```python
from build123d import *

# Parameters (mm, degrees)
F1_DEPTH = 17.5
F3_DEPTH = 15
F4_R     = 2
F5_SIZE  = 1
F7_DEPTH = 2.5
F8_R     = 1.5
F9_DEPTH = 2.5


with BuildPart() as f1:
    # F0 (on Right) → F1 (new body, symmetric)
    with BuildSketch(Plane.YZ):
        Polygon((-5, -15), (0, -15), (0, 0), (-13.9, 0), (-13.9, -15), (-10.9, -15), (-10.9, -3), (-5, -3), align=None)
    extrude(amount=F1_DEPTH, both=True)

    # F2 (on face) → F3 (join)
    with BuildSketch(Plane.XY):
        with BuildLine():
            Line((0, 0), (3.4641016151, 0))
            ThreePointArc((3.4641016151, 0), (2.2943057454, 5.2766081772), (-3.0641777725, 4.5711504387))
            ThreePointArc((-3.0641777725, 4.5711504387), (-2.940920939, 3.1623183859), (-1.5320888862, 3.2855752194))
            ThreePointArc((-1.5320888862, 3.2855752194), (1.8126155741, 2.8452365235), (0, 0))
        make_face()
        with BuildLine():
            Line((-3.4641016151, 0), (0, 0))
            ThreePointArc((0, 0), (-1, 0.2679491924), (-1.7320508076, 1))
            Line((-1.7320508076, 1), (-3.4641016151, 0))
        make_face()
    extrude(amount=-F3_DEPTH)

    # F4
    f4_edges = [f1.edges().sort_by_distance(p)[0] for p in [
        (3.464102, 0, -7.5),
        (-3.464102, 0, -7.5),
    ]]
    fillet(f4_edges, radius=F4_R)

    # F5
    f5_edges = [f1.edges().sort_by_distance(p)[0] for p in [
        (-17.5, 0, -7.5),
        (17.5, 0, -7.5),
        (-17.5, -13.9, -7.5),
        (17.5, -13.9, -7.5),
    ]]
    chamfer(f5_edges, length=F5_SIZE)

    # F6 (on face) → F7 (cut)
    with BuildSketch(Plane.XZ.offset(5)):
        Polygon((-12.5588457268, -11.7), (-9.4411542732, -11.7), (-7.8823085464, -9), (-9.4411542732, -6.3), (-12.5588457268, -6.3), (-14.1176914536, -9), align=None)
        Polygon((9.4411542732, -11.7), (12.5588457268, -11.7), (14.1176914536, -9), (12.5588457268, -6.3), (9.4411542732, -6.3), (7.8823085464, -9), align=None)
    extrude(amount=-F7_DEPTH, mode=Mode.SUBTRACT)

    # F8 (on face) → F9 (cut, through all)
    with BuildSketch(Plane(origin=(0, 0, 0), x_dir=(-1, 0, 0), z_dir=(0, 1, 0))):
        with Locations((-11, -9)):
            Circle(F8_R)
        with Locations((11, -9)):
            Circle(F8_R)
    extrude(amount=-F9_DEPTH, mode=Mode.SUBTRACT)


solid = f1.part
```
Work out the finished part from the listing and answer in its coordinate system (mm). A direction names the side the tool comes from. Give positions to 0.01 mm unless a question says otherwise; leave off trailing zeros. Write each loop counter-clockwise with the first axis right and the second up, starting at its lowest first coordinate (ties: lowest second). Pieces come first, ordered by that corner, then holes. Notation, with made-up numbers: (37.25, 39) -> (64.25, 39) arc R21 ccw to (64.25, 64) -> close; hole circle Ø11 at (78, -3.75). An arc over 180 degrees is marked (long way). Write each question's results on one line, items separated by ' | '.
1. Straight lines are drawn through the part: L1, parallel to Z at x = -11, y = -1.1; L2, parallel to Y at x = -7.5, z = -7.75; L3, parallel to Y at x = -0.5, z = -6.75. For each, find the intervals that lie inside material, in ascending order.
Data:
L1: -15 to -10.5, -7.5 to 0 | L2: -13.9 to -10.9, -5 to 0 | L3: -13.9 to -10.9, -5 to 0.06, 3.94 to 5.97
2. Find section B-B on z = -13. Determine the outline of the cut face in (x, y), and give its area (3 significant figures).
Data:
outline: (-17.5, -12.9) -> (-16.5, -13.9) -> (16.5, -13.9) -> (17.5, -12.9) -> (17.5, -10.9) -> (-17.5, -10.9) -> close; (-17.5, -5) -> (17.5, -5) -> (17.5, -1) -> (16.5, 0) -> (6, 0) arc R2 cw to (4, 2) arc R4 ccw to (-3.06, 4.57) arc R1 ccw to (-1.53, 3.29) arc R2 cw (long way) to (-1.73, 1) -> (-3, 0.27) arc R2 cw to (-4, 0) -> (-16.5, 0) -> (-17.5, -1) -> close | area: 301 mm^2
3. A tool of negligible diameter and unlimited length cuts with its end or side. For faces 1 (the flat face through (-17, -0.5, -7.6)), 2 (the cylindrical face through (-9.8, -1.2, -9.9)), 3 (the cylindrical face through (-3.489, 0.066, -7.605)), 4 (the flat face through (11, -4, -11.7)), from which of +Z, -Z, +X, -X, +Y, -Y can it reach the whole face along a straight path? Write none if from no direction.
Data:
face 1: +Z, -Z, -X, +Y | face 2: +Y | face 3: +Z, -Z, -X | face 4: none
4. Determine the mould class of faces 5 (the flat face through (0, -12, -15)), 6 (the flat face through (8.65, -3.77, -10.33)), 7 (the flat face through (-9, 0, -8)) for opening direction Z: +Z half, -Z half, draft (parallel to the pull), parting line (faces both ways), or undercut.
Data:
face 5: -Z half | face 6: undercut | face 7: draft
5. Find section A-A on x = -11. Determine the outline of the cut face in (y, z).
Data:
outline: (-13.9, -15) -> (-10.9, -15) -> (-10.9, -3) -> (-5, -3) -> (-5, -6.3) -> (-2.5, -6.3) -> (-2.5, -7.5) -> (0, -7.5) -> (0, 0) -> (-13.9, 0) -> close; (-5, -15) -> (0, -15) -> (0, -10.5) -> (-2.5, -10.5) -> (-2.5, -11.7) -> (-5, -11.7) -> close
6. This flat-tipped pin is pushed along its axis until it touches: pin 1 Ø4 at (x, z) = (-11, -9) entering from +Y. Where does it stop, or does it pass through?
Data:
pin 1: y = 0
7. Find section D-D on x = -6.5. Determine the outline of the cut face in (y, z), and give its area (3 significant figures).
Data:
outline: (-13.9, -15) -> (-10.9, -15) -> (-10.9, -3) -> (-5, -3) -> (-5, -15) -> (0, -15) -> (0, 0) -> (-13.9, 0) -> close | area: 138 mm^2
8. Find section C-C on y = -1.5. Determine the outline of the cut face in (x, z).
Data:
outline: (-17.5, -15) -> (17.5, -15) -> (17.5, 0) -> (-17.5, 0) -> close; hole circle Ø3 at (-11, -9); hole circle Ø3 at (11, -9)
